from build123d import *

# Parameters (mm, degrees)
SKETCH1_W           = 160
SKETCH1_H           = 100
BOSS_EXTRUDE1_DEPTH = 30
SKETCH2_R           = 40
BOSS_EXTRUDE2_DEPTH = 110
BOSS_EXTRUDE3_DEPTH = 100
CUT_EXTRUDE1_DEPTH  = 100
SKETCH6_W           = 60
SKETCH6_H           = 100
CUT_EXTRUDE2_DEPTH  = 1
SKETCH7_W           = 60
SKETCH7_H           = 10
CUT_EXTRUDE3_DEPTH  = 100
SKETCH8_R           = 7.5
CUT_EXTRUDE4_DEPTH  = 100


with BuildPart() as part:
    # Sketch1 → Boss-Extrude1 (new body)
    with BuildSketch(Plane(origin=(0, 0, 0), x_dir=(1, 0, 0), z_dir=(0, 1, 0))):
        with Locations((7.145359019, 50)):
            Rectangle(SKETCH1_W, SKETCH1_H)
    extrude(amount=-BOSS_EXTRUDE1_DEPTH)

    # Sketch2 → Boss-Extrude2 (add)
    with BuildSketch(Plane(origin=(0, 0, 0), x_dir=(1, 0, 0), z_dir=(0, 1, 0))):
        with Locations(Location((7.145359019, 50, 0), (0, 0, 270))):
            Circle(SKETCH2_R)
    extrude(amount=BOSS_EXTRUDE2_DEPTH)

    # Sketch3 → Boss-Extrude3 (add)
    with BuildSketch(Plane.XY):
        with BuildLine():
            Line((-37.620353567, 110), (52.379646433, 110))
            ThreePointArc((52.379646433, 110), (7.379646433, 65), (-37.620353567, 110))
        make_face()
        with BuildLine():
            Line((-22.620353567, 109.466218226), (37.379646433, 109.466218226))
            ThreePointArc((37.379646433, 109.466218226), (7.379646433, 79.466218226), (-22.620353567, 109.466218226))
        make_face(mode=Mode.SUBTRACT)
    extrude(amount=-BOSS_EXTRUDE3_DEPTH)

    # Sketch4 → Cut-Extrude1 (cut)
    with BuildSketch(Plane.XY):
        with BuildLine():
            Line((-22.620353567, 109.466218226), (37.379646433, 109.466218226))
            ThreePointArc((37.379646433, 109.466218226), (7.379646433, 79.466218226), (-22.620353567, 109.466218226))
        make_face()
    extrude(amount=-CUT_EXTRUDE1_DEPTH, mode=Mode.SUBTRACT)

    # Sketch6 → Cut-Extrude2 (cut)
    with BuildSketch(Plane(origin=(0, 110, 0), x_dir=(1, 0, 0), z_dir=(0, 1, 0))):
        with Locations((7.379646433, 50)):
            Rectangle(SKETCH6_W, SKETCH6_H)
    extrude(amount=-CUT_EXTRUDE2_DEPTH, mode=Mode.SUBTRACT)

    # Sketch7 → Cut-Extrude3 (cut)
    with BuildSketch(Plane.XY):
        with Locations((7.145359019, -25)):
            Rectangle(SKETCH7_W, SKETCH7_H)
    extrude(amount=-CUT_EXTRUDE3_DEPTH, mode=Mode.SUBTRACT)

    # Sketch8 → Cut-Extrude4 (cut)
    with BuildSketch(Plane(origin=(0, 0, 0), x_dir=(1, 0, 0), z_dir=(0, 1, 0))):
        with Locations(Location((77.145359019, 90, 0), (0, 0, 270))):
            Circle(SKETCH8_R)
        with Locations(Location((-62.854640981, 90, 0), (0, 0, 270))):
            Circle(SKETCH8_R)
        with Locations(Location((-62.854640981, 10, 0), (0, 0, 270))):
            Circle(SKETCH8_R)
        with Locations(Location((77.145359019, 10, 0), (0, 0, 270))):
            Circle(SKETCH8_R)
    extrude(amount=-CUT_EXTRUDE4_DEPTH, mode=Mode.SUBTRACT)


solid = part.part
The listing builds one solid part. Answer for the finished solid, in the listing's coordinates (mm). A direction names the side the tool comes from. Give positions to 0.01 mm unless a question says otherwise; leave off trailing zeros. Order: outer loops, then holes, each group sorted by start corner. A loop starts at its lowest first (then second) coordinate and runs counter-clockwise, first axis right, second up. Notation, with made-up numbers: (51.5, 67.5) - (104.5, 67.5) arc R20 cw to (104.5, 89.5) - close; hole circle Ø9 at (89, 5.5). An arc over 180 degrees is marked (long way). Answer as CSV lines item,"result".
Q1. A cutting plane is placed at A-A, the plane z = -12.5. Count the separate pieces of the cut face and the enclosed holes in it, and give its area (3 significant figures).
Answer key:
separate pieces,"3"
enclosed holes,"0"
area,"6,920 mm^2"
Q2. Which of the six approach directions +Z, -Z, +X, -X, +Y, -Y give full straight-line access (tool end or side, diameter ignored) to faces 4 (the face through (19.16, 34.311, -11.847)), 5 (the face through (6, -15, -100)), 6 (the face through (37.145, -25, -49))?
Answer key:
face 4,"none"
face 5,"-Z, +X, -X, +Y, -Y"
face 6,"+Z, -Z, -Y"
Q3. Determine the mould class of faces 1 (the face through (-30, 0, -28)), 2 (the face through (-22.855, -25, -49)), 3 (the face through (-30, 110, -49)) for opening direction Y: pulls with the +Y half, pulls with the -Y half, needs draft (parallel to the pull), parting line crosses it, or undercut.
Answer key:
face 1,"undercut"
face 2,"needs draft"
face 3,"pulls with the +Y half"
Q4. Straight lines are drawn through the part: L1, parallel to X at y = -12, z = -90; L2, parallel to Y at x = -59.5, z = -52; L3, parallel to Z at x = 9, y = 37. For each, find the intervals that lie inside material, in ascending order.
Answer key:
L1,"x = -72.85 to -70.35, -55.35 to 69.65, 84.65 to 87.15"
L2,"y = -30 to 0"
L3,"z = -89.96 to -10.04"
Q5. A cutting plane is placed at B-B, the plane y = -2.5. Determine the outline of the cut face in (x, z).
Answer key:
outline,"(-72.85, -100) - (87.15, -100) - (87.15, 0) - (-72.85, 0) - close; hole circle Ø15 at (-62.85, -90); hole circle Ø15 at (-62.85, -10); hole circle Ø15 at (77.15, -90); hole circle Ø15 at (77.15, -10)"
Q6. Each of these flat-tipped pins is pushed along its axis until it touches: pin 1 Ø13.5 at (x, z) = (77.15, -10) entering from -Y; pin 2 Ø6 at (x, z) = (30.5, -57) entering from +Y; pin 3 Ø1 at (y, z) = (44, -65.5) entering from -X; pin 4 Ø0.5 at (y, z) = (109.5, -74) entering from +X. Where does it stop, or does it pass through?
Answer key:
pin 1,"passes through"
pin 2,"stops at y = 94.71"
pin 3,"stops at x = -29.94"
pin 4,"stops at x = 52.38"
